Input: part model. Units: mm. Frame: model coordinates. A direction names the side the tool comes from. Round coordinates to 2 decimals unless told otherwise and drop trailing zeros. Order: outer loops, then holes, each group sorted by start corner. A loop starts at its lowest first (then second) coordinate and runs counter-clockwise, first axis right, second up. Notation, with made-up numbers: (7, 60) - (29, 60) arc R29 cw to (29, 83) - close; hole circle Ø1 at (-14, 37). An arc over 180 degrees is marked (long way). One line per item, written item: value. Start each with the question number.
from build123d import *

# Parameters (mm, degrees)
F3_D     = 4.2
F3_DEPTH = 12
F3_TIP   = 1.2618073
F5_DEPTH = 13.6086951546


with BuildPart() as f1:
    # F0 (on Front) → F1 (revolve)
    with BuildSketch(Plane.XZ):
        with BuildLine():
            Line((-6, 12), (-6, 0))
            Line((-6, 0), (0, 0))
            Line((0, 0), (0, 13.6076951546))
            ThreePointArc((0, 13.6076951546), (-3.1058285412, 13.1988050701), (-6, 12))
        make_face()
    revolve(axis=Axis((0, 0, 6.8038475773), (0, 0, -1)))

    # F3
    with Locations(Plane(origin=(0, 0, 0), x_dir=(1, 0, 0), z_dir=(0, 0, -1))):
        with Locations((0, 0)):
            Hole(F3_D / 2, depth=F3_DEPTH)
            with Locations((0, 0, -(F3_DEPTH + F3_TIP / 2))):  # 118° drill point
                Cone(0, F3_D / 2, F3_TIP, mode=Mode.SUBTRACT)

    # F4 (on Top) → F5 (intersect, through all)
    with BuildSketch(Plane.XY):
        Polygon((-2.897095172, 4.9940137062), (-5.7734903224, -0.011951163), (-2.8763951504, -5.0059648692), (2.897095172, -4.9940137062), (5.7734903224, 0.011951163), (2.8763951504, 5.0059648692), align=None)
    extrude(amount=F5_DEPTH, mode=Mode.INTERSECT)


solid = f1.part
Item 1: Section query B-B on y = 3.25. Return loops of the section in (x, z).
Item 2: Line query: L1, parallel to Y at x = -0.5, z = 7.25; L2, parallel to Y at x = 0, z = 7.5; L3, parallel to X at y = -1.5, z = 1.25. Output: solid intervals per line, ascending.
Item 3: Pull-direction query (Y, two-part tool) for faces 3 (the face through (4.345, 2.474, 6.171)), 4 (the face through (0.35, -0.11, 13.04)), 5 (the face through (-2.5, 0.1, 0)); classes: released by +Y, released by -Y, zero draft, split by the parting line, or undercut.
Item 4: Section query A-A on z = 3. Return loops of the section in (x, y), and give its area (3 significant figures).
Item 5: Section query C-C on x = -4.75. Return loops of the section in (y, z), and give its area (3 significant figures).
Item 6: First-contact query: pin 1 Ø1 at (y, z) = (-1.5, 9.5) entering from +X; pin 2 Ø3 at (x, z) = (-3, 9.5) entering from +Y; pin 3 Ø1 at (x, z) = (1.5, 12) entering from -Y. Flat tips, straight axial feed; report the tip coordinate or a pass-through.
Item 7: Reachability of faces 1 (the face through (-2.003, -0.631, 6.084)), 2 (the face through (4.315, -2.526, 6.171)) from +Z, -Z, +X, -X, +Y, -Y: full face, straight path, thin tool, end or side. Return the list, or none.
Geometry results:
1. outline: (-3.9, 0) - (3.9, 0) - (3.9, 12.48) arc R11.55 ccw to (-3.9, 12.48) - close
2. L1: y = -5 to -2.04, 2.04 to 5
2. L2: y = -5 to -2.1, 2.1 to 5
2. L3: x = -4.91 to -1.47, 1.47 to 4.9
3. face 3: released by +Y
3. face 4: undercut
3. face 5: zero draft
4. outline: (-5.77, -0.01) - (-2.88, -5.01) - (2.9, -4.99) - (5.77, 0.01) - (2.88, 5.01) - (-2.9, 4.99) - close; hole circle Ø4.2 at (0, 0)
4. area: 72.7 mm^2
5. outline: (-1.78, 0) - (1.77, 0) - (1.77, 12.48) arc R11.02 ccw to (-1.78, 12.48) - close
5. area: 44.6 mm^2
6. pin 1: stops at x = 5.19
6. pin 2: stops at y = 5
6. pin 3: stops at y = -5
7. face 1: -Z
7. face 2: +Z, -Z, +X, -Y
